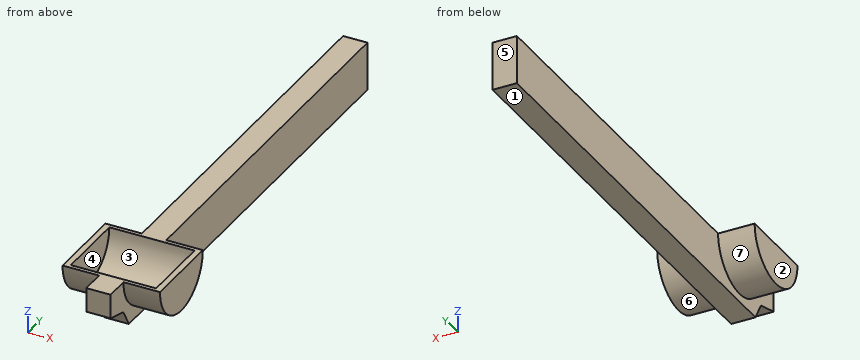
from build123d import *

# Parameters (mm, degrees)
F0_W     = 19.05
F0_H     = 38.1
F1_DEPTH = 190.5
F3_DEPTH = 38.1
F6_W     = 66.675
F6_H     = 28.575
F9_DEPTH = 47.626


with BuildPart() as f1:
    # F0 (on Front) → F1 (new body, symmetric)
    with BuildSketch(Plane.XZ):
        Rectangle(F0_W, F0_H)
    extrude(amount=F1_DEPTH, both=True)

    # F2 (on Right) → F3 (join, symmetric)
    with BuildSketch(Plane.YZ):
        with BuildLine():
            Line((-107.95, 19.05), (-171.45, 19.05))
            ThreePointArc((-171.45, 19.05), (-139.7, -12.7), (-107.95, 19.05))
        make_face()
    extrude(amount=F3_DEPTH, both=True)

    # F6 (on face) → F7 (revolve, cut)
    with BuildSketch(Plane.XY.offset(19.05)):
        with Locations((0, -125.4125)):
            Rectangle(F6_W, F6_H)
    revolve(axis=Axis((58.379408, -139.7, 19.05), (1, 0, 0)), mode=Mode.SUBTRACT)

    # F8 (on face) → F9 (cut, through all)
    with BuildSketch(Plane.YZ.offset(9.525)):
        Polygon((-171.45, -5.197727), (-190.5, 0), (-190.5, -19.05), (-163.452387, -19.05), align=None)
    extrude(amount=-F9_DEPTH, mode=Mode.SUBTRACT)


solid = f1.part
The model under review builds one solid part; all positions refer to its coordinate system, in mm. Face numbers are marked on the shaded views. A direction names the side the tool comes from. Coordinates: 2 decimals unless noted, no trailing zeros. Order: outer loops, then holes, each group sorted by start corner. A loop starts at its lowest first (then second) coordinate and runs counter-clockwise, first axis right, second up. Notation, with made-up numbers: (-10, -9) -> (34, -9) arc R11 cw to (34, 4) -> close; hole circle Ø3 at (82.5, 84.5). An arc over 180 degrees is marked (long way). Answer in a Markdown table with one row per item.
(1) Machinability: for the marked faces 5, 6 and 7, which of the approach directions +Z, -Z, +X, -X, +Y, -Y give a long, thin tool a straight path to every point of the face, cutting with its end or side? Answer none if there is none.
Answers:
| item | result |
|---|---|
| face 5 | +Z, -Z, +X, -X, +Y |
| face 6 | -Z, +X |
| face 7 | -Z, -X |
(2) The part is to be moulded in two halves that separate along X. For the marked faces 1, 2, 3 and 4, say which applies: +X half, -X half, draft (parallel to the pull), parting line (faces both ways), or undercut.
Answers:
| item | result |
|---|---|
| face 1 | draft |
| face 2 | -X half |
| face 3 | undercut |
| face 4 | undercut |
(3) Wall thickness on line 1 along X through (y, z) = (-154.5, 1); line 2 along X through (y, z) = (63, 10.5) (3 decimals); line 3 along Y through (x, z) = (3.5, 2.5): over which ranges is each line inside the solid? List them lowest first.
Answers:
| item | result |
|---|---|
| line 1 | -38.1 to -33.34, 33.34 to 38.1 |
| line 2 | -9.525 to 9.525 |
| line 3 | -190.5 to -162.99, -116.41 to 190.5 |
(4) Consider section D-D (y = -30). Write out the cut boundary in (x, z) (3 decimals).
Answers:
| item | result |
|---|---|
| outline | (-9.525, -19.05) -> (9.525, -19.05) -> (9.525, 19.05) -> (-9.525, 19.05) -> close |
(5) Consider section B-B (x = 1.5). Write out the cut boundary in (y, z) (3 decimals).
Answers:
| item | result |
|---|---|
| outline | (-190.5, 0) -> (-171.45, -5.198) -> (-163.452, -19.05) -> (190.5, -19.05) -> (190.5, 19.05) -> (-111.125, 19.05) arc R28.575 cw to (-168.275, 19.05) -> (-190.5, 19.05) -> close |
(6) Consider section A-A (z = 14.5). Write out the cut boundary in (x, y) (1 decimal), plus the area to 3 significant figures.
Answers:
| item | result |
|---|---|
| outline | (-38.1, -171.1) -> (-9.5, -171.1) -> (-9.5, -190.5) -> (9.5, -190.5) -> (9.5, -171.1) -> (38.1, -171.1) -> (38.1, -108.3) -> (9.5, -108.3) -> (9.5, 190.5) -> (-9.5, 190.5) -> (-9.5, -108.3) -> (-38.1, -108.3) -> close; hole (-33.3, -167.9) -> (33.3, -167.9) -> (33.3, -111.5) -> (-33.3, -111.5) -> close |
| area | 7,090 mm² |
(7) Insertion check: pin 1 (5 mm diameter, centred on y = 137, z = -1, fed in from +X) (3 decimals); pin 2 (5 mm diameter, centred on y = -44, z = 13.5, fed in from -X) (3 decimals); pin 3 (2 mm diameter, centred on x = -21, z = 14, fed in from +Y); pin 4 (2 mm diameter, centred on x = -17, z = -15, fed in from -Y). Each pin has a flat end and moves straight along its axis. Give the tip position at first contact, or say it passes through.
Answers:
| item | result |
|---|---|
| pin 1 | x = 9.525 |
| pin 2 | x = -9.525 |
| pin 3 | y = -108.21 |
| pin 4 | through |
